from build123d import *

# Parameters (mm, degrees)
TPS_SILIKON_GN21_20_CUKUR_1_START  = 9
SKETCH1_W                          = 530
SKETCH1_H                          = 650
TPS_SILIKON_GN21_20_CUKUR_1_DEPTH  = 30
TPS_SILIKON_GN21_20_CUKUR_2_START  = 19
SKETCH2_R                          = 60
TPS_SILIKON_GN21_20_CUKUR_2_DEPTH  = 21
TPS_SILIKON_GN21_20_CUKUR_3_START  = 19
SKETCH3_R                          = 60
TPS_SILIKON_GN21_20_CUKUR_3_DEPTH  = 21
TPS_SILIKON_GN21_20_CUKUR_4_START  = 19
SKETCH4_R                          = 60
TPS_SILIKON_GN21_20_CUKUR_4_DEPTH  = 21
TPS_SILIKON_GN21_20_CUKUR_5_START  = 19
SKETCH5_R                          = 60
TPS_SILIKON_GN21_20_CUKUR_5_DEPTH  = 21
TPS_SILIKON_GN21_20_CUKUR_6_START  = 19
SKETCH6_R                          = 60
TPS_SILIKON_GN21_20_CUKUR_6_DEPTH  = 21
TPS_SILIKON_GN21_20_CUKUR_7_START  = 19
SKETCH7_R                          = 60
TPS_SILIKON_GN21_20_CUKUR_7_DEPTH  = 21
TPS_SILIKON_GN21_20_CUKUR_8_START  = 19
SKETCH8_R                          = 60
TPS_SILIKON_GN21_20_CUKUR_8_DEPTH  = 21
TPS_SILIKON_GN21_20_CUKUR_9_START  = 19
SKETCH9_R                          = 60
TPS_SILIKON_GN21_20_CUKUR_9_DEPTH  = 21
TPS_SILIKON_GN21_20_CUKUR_10_START = 19
SKETCH10_R                         = 60
TPS_SILIKON_GN21_20_CUKUR_10_DEPTH = 21
TPS_SILIKON_GN21_20_CUKUR_11_START = 19
SKETCH11_R                         = 60
TPS_SILIKON_GN21_20_CUKUR_11_DEPTH = 21
TPS_SILIKON_GN21_20_CUKUR_12_START = 19
SKETCH12_R                         = 60
TPS_SILIKON_GN21_20_CUKUR_12_DEPTH = 21
TPS_SILIKON_GN21_20_CUKUR_13_START = 19
SKETCH13_R                         = 60
TPS_SILIKON_GN21_20_CUKUR_13_DEPTH = 21
TPS_SILIKON_GN21_20_CUKUR_14_START = 19
SKETCH14_R                         = 60
TPS_SILIKON_GN21_20_CUKUR_14_DEPTH = 21
TPS_SILIKON_GN21_20_CUKUR_15_START = 19
SKETCH15_R                         = 60
TPS_SILIKON_GN21_20_CUKUR_15_DEPTH = 21
TPS_SILIKON_GN21_20_CUKUR_16_START = 19
SKETCH16_R                         = 60
TPS_SILIKON_GN21_20_CUKUR_16_DEPTH = 21
TPS_SILIKON_GN21_20_CUKUR_17_START = 19
SKETCH17_R                         = 60
TPS_SILIKON_GN21_20_CUKUR_17_DEPTH = 21
TPS_SILIKON_GN21_20_CUKUR_18_START = 19
SKETCH18_R                         = 60
TPS_SILIKON_GN21_20_CUKUR_18_DEPTH = 21
TPS_SILIKON_GN21_20_CUKUR_19_START = 19
SKETCH19_R                         = 60
TPS_SILIKON_GN21_20_CUKUR_19_DEPTH = 21
TPS_SILIKON_GN21_20_CUKUR_20_START = 19
SKETCH20_R                         = 60
TPS_SILIKON_GN21_20_CUKUR_20_DEPTH = 21
TPS_SILIKON_GN21_20_CUKUR_21_START = 19
SKETCH21_R                         = 60
TPS_SILIKON_GN21_20_CUKUR_21_DEPTH = 21


with BuildPart() as part:
    # Sketch1 → TPS_silikon_GN21_20_cukur_1 (new body)
    with BuildSketch(Plane(origin=(0, 0, 0), x_dir=(1, 0, 0), z_dir=(0, 1, 0)).offset(TPS_SILIKON_GN21_20_CUKUR_1_START)):
        with Locations((309, 350)):
            Rectangle(SKETCH1_W, SKETCH1_H)
    extrude(amount=TPS_SILIKON_GN21_20_CUKUR_1_DEPTH)

    # Sketch2 → TPS_silikon_GN21_20_cukur_2 (cut)
    with BuildSketch(Plane(origin=(0, 0, 0), x_dir=(1, 0, 0), z_dir=(0, 1, 0)).offset(TPS_SILIKON_GN21_20_CUKUR_2_START)):
        with Locations(Location((114, 610, 0), (0, 0, 90))):
            Circle(SKETCH2_R)
    extrude(amount=TPS_SILIKON_GN21_20_CUKUR_2_DEPTH, mode=Mode.SUBTRACT)

    # Sketch3 → TPS_silikon_GN21_20_cukur_3 (cut)
    with BuildSketch(Plane(origin=(0, 0, 0), x_dir=(1, 0, 0), z_dir=(0, 1, 0)).offset(TPS_SILIKON_GN21_20_CUKUR_3_START)):
        with Locations(Location((114, 480, 0), (0, 0, 90))):
            Circle(SKETCH3_R)
    extrude(amount=TPS_SILIKON_GN21_20_CUKUR_3_DEPTH, mode=Mode.SUBTRACT)

    # Sketch4 → TPS_silikon_GN21_20_cukur_4 (cut)
    with BuildSketch(Plane(origin=(0, 0, 0), x_dir=(1, 0, 0), z_dir=(0, 1, 0)).offset(TPS_SILIKON_GN21_20_CUKUR_4_START)):
        with Locations(Location((114, 350, 0), (0, 0, 90))):
            Circle(SKETCH4_R)
    extrude(amount=TPS_SILIKON_GN21_20_CUKUR_4_DEPTH, mode=Mode.SUBTRACT)

    # Sketch5 → TPS_silikon_GN21_20_cukur_5 (cut)
    with BuildSketch(Plane(origin=(0, 0, 0), x_dir=(1, 0, 0), z_dir=(0, 1, 0)).offset(TPS_SILIKON_GN21_20_CUKUR_5_START)):
        with Locations(Location((114, 220, 0), (0, 0, 90))):
            Circle(SKETCH5_R)
    extrude(amount=TPS_SILIKON_GN21_20_CUKUR_5_DEPTH, mode=Mode.SUBTRACT)

    # Sketch6 → TPS_silikon_GN21_20_cukur_6 (cut)
    with BuildSketch(Plane(origin=(0, 0, 0), x_dir=(1, 0, 0), z_dir=(0, 1, 0)).offset(TPS_SILIKON_GN21_20_CUKUR_6_START)):
        with Locations(Location((114, 90, 0), (0, 0, 90))):
            Circle(SKETCH6_R)
    extrude(amount=TPS_SILIKON_GN21_20_CUKUR_6_DEPTH, mode=Mode.SUBTRACT)

    # Sketch7 → TPS_silikon_GN21_20_cukur_7 (cut)
    with BuildSketch(Plane(origin=(0, 0, 0), x_dir=(1, 0, 0), z_dir=(0, 1, 0)).offset(TPS_SILIKON_GN21_20_CUKUR_7_START)):
        with Locations(Location((244, 610, 0), (0, 0, 90))):
            Circle(SKETCH7_R)
    extrude(amount=TPS_SILIKON_GN21_20_CUKUR_7_DEPTH, mode=Mode.SUBTRACT)

    # Sketch8 → TPS_silikon_GN21_20_cukur_8 (cut)
    with BuildSketch(Plane(origin=(0, 0, 0), x_dir=(1, 0, 0), z_dir=(0, 1, 0)).offset(TPS_SILIKON_GN21_20_CUKUR_8_START)):
        with Locations(Location((244, 480, 0), (0, 0, 90))):
            Circle(SKETCH8_R)
    extrude(amount=TPS_SILIKON_GN21_20_CUKUR_8_DEPTH, mode=Mode.SUBTRACT)

    # Sketch9 → TPS_silikon_GN21_20_cukur_9 (cut)
    with BuildSketch(Plane(origin=(0, 0, 0), x_dir=(1, 0, 0), z_dir=(0, 1, 0)).offset(TPS_SILIKON_GN21_20_CUKUR_9_START)):
        with Locations(Location((244, 350, 0), (0, 0, 90))):
            Circle(SKETCH9_R)
    extrude(amount=TPS_SILIKON_GN21_20_CUKUR_9_DEPTH, mode=Mode.SUBTRACT)

    # Sketch10 → TPS_silikon_GN21_20_cukur_10 (cut)
    with BuildSketch(Plane(origin=(0, 0, 0), x_dir=(1, 0, 0), z_dir=(0, 1, 0)).offset(TPS_SILIKON_GN21_20_CUKUR_10_START)):
        with Locations(Location((244, 220, 0), (0, 0, 90))):
            Circle(SKETCH10_R)
    extrude(amount=TPS_SILIKON_GN21_20_CUKUR_10_DEPTH, mode=Mode.SUBTRACT)

    # Sketch11 → TPS_silikon_GN21_20_cukur_11 (cut)
    with BuildSketch(Plane(origin=(0, 0, 0), x_dir=(1, 0, 0), z_dir=(0, 1, 0)).offset(TPS_SILIKON_GN21_20_CUKUR_11_START)):
        with Locations(Location((244, 90, 0), (0, 0, 90))):
            Circle(SKETCH11_R)
    extrude(amount=TPS_SILIKON_GN21_20_CUKUR_11_DEPTH, mode=Mode.SUBTRACT)

    # Sketch12 → TPS_silikon_GN21_20_cukur_12 (cut)
    with BuildSketch(Plane(origin=(0, 0, 0), x_dir=(1, 0, 0), z_dir=(0, 1, 0)).offset(TPS_SILIKON_GN21_20_CUKUR_12_START)):
        with Locations(Location((374, 610, 0), (0, 0, 90))):
            Circle(SKETCH12_R)
    extrude(amount=TPS_SILIKON_GN21_20_CUKUR_12_DEPTH, mode=Mode.SUBTRACT)

    # Sketch13 → TPS_silikon_GN21_20_cukur_13 (cut)
    with BuildSketch(Plane(origin=(0, 0, 0), x_dir=(1, 0, 0), z_dir=(0, 1, 0)).offset(TPS_SILIKON_GN21_20_CUKUR_13_START)):
        with Locations(Location((374, 480, 0), (0, 0, 90))):
            Circle(SKETCH13_R)
    extrude(amount=TPS_SILIKON_GN21_20_CUKUR_13_DEPTH, mode=Mode.SUBTRACT)

    # Sketch14 → TPS_silikon_GN21_20_cukur_14 (cut)
    with BuildSketch(Plane(origin=(0, 0, 0), x_dir=(1, 0, 0), z_dir=(0, 1, 0)).offset(TPS_SILIKON_GN21_20_CUKUR_14_START)):
        with Locations(Location((374, 350, 0), (0, 0, 90))):
            Circle(SKETCH14_R)
    extrude(amount=TPS_SILIKON_GN21_20_CUKUR_14_DEPTH, mode=Mode.SUBTRACT)

    # Sketch15 → TPS_silikon_GN21_20_cukur_15 (cut)
    with BuildSketch(Plane(origin=(0, 0, 0), x_dir=(1, 0, 0), z_dir=(0, 1, 0)).offset(TPS_SILIKON_GN21_20_CUKUR_15_START)):
        with Locations(Location((374, 220, 0), (0, 0, 90))):
            Circle(SKETCH15_R)
    extrude(amount=TPS_SILIKON_GN21_20_CUKUR_15_DEPTH, mode=Mode.SUBTRACT)

    # Sketch16 → TPS_silikon_GN21_20_cukur_16 (cut)
    with BuildSketch(Plane(origin=(0, 0, 0), x_dir=(1, 0, 0), z_dir=(0, 1, 0)).offset(TPS_SILIKON_GN21_20_CUKUR_16_START)):
        with Locations(Location((374, 90, 0), (0, 0, 90))):
            Circle(SKETCH16_R)
    extrude(amount=TPS_SILIKON_GN21_20_CUKUR_16_DEPTH, mode=Mode.SUBTRACT)

    # Sketch17 → TPS_silikon_GN21_20_cukur_17 (cut)
    with BuildSketch(Plane(origin=(0, 0, 0), x_dir=(1, 0, 0), z_dir=(0, 1, 0)).offset(TPS_SILIKON_GN21_20_CUKUR_17_START)):
        with Locations(Location((504, 610, 0), (0, 0, 90))):
            Circle(SKETCH17_R)
    extrude(amount=TPS_SILIKON_GN21_20_CUKUR_17_DEPTH, mode=Mode.SUBTRACT)

    # Sketch18 → TPS_silikon_GN21_20_cukur_18 (cut)
    with BuildSketch(Plane(origin=(0, 0, 0), x_dir=(1, 0, 0), z_dir=(0, 1, 0)).offset(TPS_SILIKON_GN21_20_CUKUR_18_START)):
        with Locations(Location((504, 480, 0), (0, 0, 90))):
            Circle(SKETCH18_R)
    extrude(amount=TPS_SILIKON_GN21_20_CUKUR_18_DEPTH, mode=Mode.SUBTRACT)

    # Sketch19 → TPS_silikon_GN21_20_cukur_19 (cut)
    with BuildSketch(Plane(origin=(0, 0, 0), x_dir=(1, 0, 0), z_dir=(0, 1, 0)).offset(TPS_SILIKON_GN21_20_CUKUR_19_START)):
        with Locations(Location((504, 350, 0), (0, 0, 90))):
            Circle(SKETCH19_R)
    extrude(amount=TPS_SILIKON_GN21_20_CUKUR_19_DEPTH, mode=Mode.SUBTRACT)

    # Sketch20 → TPS_silikon_GN21_20_cukur_20 (cut)
    with BuildSketch(Plane(origin=(0, 0, 0), x_dir=(1, 0, 0), z_dir=(0, 1, 0)).offset(TPS_SILIKON_GN21_20_CUKUR_20_START)):
        with Locations(Location((504, 220, 0), (0, 0, 90))):
            Circle(SKETCH20_R)
    extrude(amount=TPS_SILIKON_GN21_20_CUKUR_20_DEPTH, mode=Mode.SUBTRACT)

    # Sketch21 → TPS_silikon_GN21_20_cukur_21 (cut)
    with BuildSketch(Plane(origin=(0, 0, 0), x_dir=(1, 0, 0), z_dir=(0, 1, 0)).offset(TPS_SILIKON_GN21_20_CUKUR_21_START)):
        with Locations(Location((504, 90, 0), (0, 0, 90))):
            Circle(SKETCH21_R)
    extrude(amount=TPS_SILIKON_GN21_20_CUKUR_21_DEPTH, mode=Mode.SUBTRACT)


solid = part.part
Here's how the part is built. I have some questions about the finished solid (model axes, mm). A direction names the side the tool comes from. Coordinates: 2 decimals unless noted, no trailing zeros. Write each loop counter-clockwise with the first axis right and the second up, starting at its lowest first coordinate (ties: lowest second). Pieces come first, ordered by that corner, then holes.
Item 1: If we mould it in two halves opening along Z, with no side actions, what happens to faces 1 (the flat face through (503, 19, -89)), 2 (the flat face through (308, 39, -327))? For each: +Z half, -Z half, draft (parallel to the pull), parting line (faces both ways), or undercut.
Item 2: I want a section at B-B on x = 504. Write out the boundary of the cut face in (y, z), and give its area (3 significant figures).
Item 3: On a 3-axis mill with a long thin cutter (end or side, diameter ignored), from which of +Z, -Z, +X, -X, +Y, -Y can I reach the whole of each face in a straight line? I mean faces 3 (the flat face through (44, 24, -345)), 4 (the cylindrical face through (444.51, 28.86, -82.19)). Say none if no direction works.
Item 4: I want a section at A-A on y = 34. Count the separate pieces of the cut face and the enclosed holes in it, and give its area (3 significant figures).
Item 5: If I drill on line 1 (Z direction, x = 504, y = 24.5); line 2 (X direction, y = 29, z = -90); line 3 (Z direction, x = 538, y = 22), over which ranges is the centre line in solid material (lowest first)?
Item 6: I want a section at C-C on z = -610. Write out the boundary of the cut face in (x, y).
Item 7: I want a section at D-D on z = -138. Write out the boundary of the cut face in (x, y), and give its area (3 significant figures).
Findings below:
1. face 1: undercut
1. face 2: draft
2. outline: (9, -675) - (39, -675) - (39, -670) - (19, -670) - (19, -550) - (39, -550) - (39, -540) - (19, -540) - (19, -420) - (39, -420) - (39, -410) - (19, -410) - (19, -290) - (39, -290) - (39, -280) - (19, -280) - (19, -160) - (39, -160) - (39, -150) - (19, -150) - (19, -30) - (39, -30) - (39, -25) - (9, -25) - close
2. area: 7,500 mm2
3. face 3: +Z, -Z, -X, +Y, -Y
3. face 4: +Y
4. separate pieces: 1
4. enclosed holes: 20
4. area: 118,000 mm2
5. line 1: z = -675 to -670, -550 to -540, -420 to -410, -290 to -280, -160 to -150, -30 to -25
5. line 2: x = 44 to 54, 174 to 184, 304 to 314, 434 to 444, 564 to 574
5. line 3: z = -675 to -659.44, -560.56 to -529.44, -430.56 to -399.44, -300.56 to -269.44, -170.56 to -139.44, -40.56 to -25
6. outline: (44, 9) - (574, 9) - (574, 39) - (564, 39) - (564, 19) - (444, 19) - (444, 39) - (434, 39) - (434, 19) - (314, 19) - (314, 39) - (304, 39) - (304, 19) - (184, 19) - (184, 39) - (174, 39) - (174, 19) - (54, 19) - (54, 39) - (44, 39) - close
7. outline: (44, 9) - (574, 9) - (574, 39) - (540, 39) - (540, 19) - (468, 19) - (468, 39) - (410, 39) - (410, 19) - (338, 19) - (338, 39) - (280, 39) - (280, 19) - (208, 19) - (208, 39) - (150, 39) - (150, 19) - (78, 19) - (78, 39) - (44, 39) - close
7. area: 10,100 mm2
